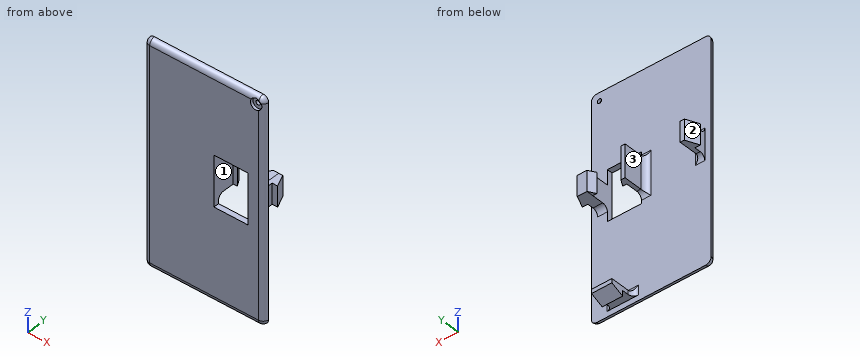
from build123d import *

# Parameters (mm, degrees)
SKETCH_1_W          = 44
SKETCH_1_H          = 81
EXTRUDE_1_DEPTH     = 2
FILLET_1_R          = 2
SKETCH_4_W          = 1.5
SKETCH_4_H          = 7.5
EXTRUDE_4_DEPTH     = 8.8
EXTRUDE_5_DEPTH     = 7.5
SKETCH_7_R          = 0.8
CUT_EXTRUDE_1_DEPTH = 8.8
SKETCH_8_R          = 2
CUT_EXTRUDE_2_DEPTH = 1
SKETCH_10_W         = 7.5
SKETCH_10_H         = 1.5
EXTRUDE_6_DEPTH     = 9
EXTRUDE_7_DEPTH     = 7.5
SKETCH_12_W         = 12.5
SKETCH_12_H         = 18.4
CUT_EXTRUDE_3_DEPTH = 7.5
SKETCH_13_W         = 2.075122626
SKETCH_13_H         = 7.498383059
EXTRUDE_8_DEPTH     = 8.8
EXTRUDE_9_DEPTH     = 7.5
SKETCH_15_W         = 1.5
SKETCH_15_H         = 12
EXTRUDE_10_DEPTH    = 8.8
EXTRUDE_11_DEPTH    = 12
FILLET_2_R          = 2


with BuildPart() as part:
    # 草图1 → 凸台-拉伸1 (new body)
    with BuildSketch(Plane(origin=(0, 0, 0), x_dir=(1, 0, 0), z_dir=(0, 1, 0))):
        with Locations((0, 2.5)):
            Rectangle(SKETCH_1_W, SKETCH_1_H)
    extrude(amount=EXTRUDE_1_DEPTH)

    # 圆角1
    fillet_1_edges = [part.edges().sort_by_distance(p)[0] for p in [
        (0, 0, -43),
        (22, 0, -2.5),
        (0, 0, 38),
        (-22, 0, -2.5),
        (-22, 1, -43),
        (22, 1, -43),
        (22, 1, 38),
        (-22, 1, 38),
    ]]
    fillet(fillet_1_edges, radius=FILLET_1_R - 0.0001)  # a hair under: the kernel refuses the full size

    # 草图4 → 凸台-拉伸4 (add)
    with BuildSketch(Plane(origin=(0, 2, 0), x_dir=(1, 0, 0), z_dir=(0, 1, 0))):
        with Locations((-18.924971335, 0)):
            Rectangle(SKETCH_4_W, SKETCH_4_H)
    extrude_4 = extrude(amount=EXTRUDE_4_DEPTH)

    # 草图6 → 凸台-拉伸5 (add)
    with BuildSketch(Plane.XY.offset(3.75)):
        Polygon((-19.674971335, 10.8), (-21.674971335, 6.2), (-19.674971335, 6.2), align=None)
    extrude_5 = extrude(amount=-EXTRUDE_5_DEPTH)

    # 镜向2: 凸台-拉伸4, 凸台-拉伸5 across plane
    add(extrude_4.mirror(Plane(origin=(0, 0, 0), x_dir=(0, 0, 1), z_dir=(1, 0, 0))))
    add(extrude_5.mirror(Plane(origin=(0, 0, 0), x_dir=(0, 0, 1), z_dir=(1, 0, 0))))

    # 草图7 → 切除-拉伸1 (cut)
    with BuildSketch(Plane.XZ):
        with Locations(Location((19, 35, 0), (0, 0, 270))):
            Circle(SKETCH_7_R)
    extrude(amount=-CUT_EXTRUDE_1_DEPTH, mode=Mode.SUBTRACT)

    # 草图8 → 切除-拉伸2 (cut)
    with BuildSketch(Plane.XZ):
        with Locations(Location((19, 35, 0), (0, 0, 270))):
            Circle(SKETCH_8_R)
    extrude(amount=-CUT_EXTRUDE_2_DEPTH, mode=Mode.SUBTRACT)

    # 草图10 → 凸台-拉伸6 (add)
    with BuildSketch(Plane(origin=(0, 2, 0), x_dir=(1, 0, 0), z_dir=(0, 1, 0))):
        with Locations((10.5, 40.25)):
            Rectangle(SKETCH_10_W, SKETCH_10_H)
    extrude(amount=EXTRUDE_6_DEPTH)

    # 草图11 → 凸台-拉伸7 (add)
    with BuildSketch(Plane(origin=(14.25, 0, 0), x_dir=(0, 0, -1), z_dir=(1, 0, 0))):
        Polygon((41, 11), (43, 6.4), (41, 6.4), align=None)
    extrude(amount=-EXTRUDE_7_DEPTH)

    # 草图12 → 切除-拉伸3 (cut)
    with BuildSketch(Plane.XZ):
        with Locations((9.849848709, 0)):
            Rectangle(SKETCH_12_W, SKETCH_12_H)
    extrude(amount=-CUT_EXTRUDE_3_DEPTH, mode=Mode.SUBTRACT)

    # 草图13 → 凸台-拉伸8 (add)
    with BuildSketch(Plane(origin=(0, 2, 0), x_dir=(1, 0, 0), z_dir=(0, 1, 0))):
        with Locations((17.137410022, 0.000808471)):
            Rectangle(SKETCH_13_W, SKETCH_13_H)
    extrude(amount=EXTRUDE_8_DEPTH)

    # 草图14 → 凸台-拉伸9 (add)
    with BuildSketch(Plane.XY.offset(3.748383059)):
        Polygon((16.099848709, 10.8), (14.599848709, 8.3), (16.099848709, 8.3), align=None)
    extrude(amount=-EXTRUDE_9_DEPTH)

    # 草图15 → 凸台-拉伸10 (add)
    with BuildSketch(Plane(origin=(0, 2, 0), x_dir=(1, 0, 0), z_dir=(0, 1, 0))):
        with Locations((2.849848709, 0)):
            Rectangle(SKETCH_15_W, SKETCH_15_H)
    extrude(amount=EXTRUDE_10_DEPTH)

    # 草图16 → 凸台-拉伸11 (add)
    with BuildSketch(Plane.XY.offset(6)):
        Polygon((3.599848709, 10.8), (5.099848709, 8.3), (3.599848709, 8.3), align=None)
    extrude(amount=-EXTRUDE_11_DEPTH)

    # 圆角2
    fillet_2_edges = [part.edges().sort_by_distance(p)[0] for p in [
        (6.75, 2, -40.25),
        (10.5, 2, -39.5),
        (14.25, 2, -40.25),
        (2.849848709, 2, -6),
        (2.099848709, 2, 0),
        (2.849848709, 2, 6),
        (-18.924971335, 2, 3.75),
        (-18.174971335, 2, 0),
        (-18.924971335, 2, -3.75),
        (17.887410022, 2, -3.75),
    ]]
    fillet(fillet_2_edges, radius=FILLET_2_R)


solid = part.part
Here's how the part is built. I have some questions about the finished solid (model axes, mm). Face numbers are marked on the shaded views. A direction names the side the tool comes from. Round coordinates to 2 decimals unless told otherwise and drop trailing zeros. Write each question's results on one line, items separated by ' | '. Start each with the question number.
(1) If I drill on probe 1 along X at (y, z) = (9.75, -2); probe 2 along Y at (x, z) = (0, 8); probe 3 along Z at (x, y) = (-19, 4.75), over which ranges is the centre line in solid material (lowest first)? Write a range as from..to.
(2) Will these pins go through, and if not, where does the flat tip stop? P1, Ø1.8, axis at x = -20, y = 6, coming from the +Z side; P2, Ø1, axis at y = 8.5, z = -7, coming from the +X side; P3, Ø2, axis at x = 2, y = 7, coming from the +Z side; P4, Ø2, axis at y = 4, z = 0.5, coming from the +X side (3 decimals).
(3) On a 3-axis mill with a long thin cutter (end or side, diameter ignored), from which of +Z, -Z, +X, -X, +Y, -Y can I reach the whole of each face in a straight line? I mean the marked faces 1, 2 and 3. Say none if no direction works.
Solved:
1) probe 1: x = -20.13..-18.17, 2.1..4.23, 15.47..20.13 | probe 2: y = 0..2 | probe 3: z = -3.75..3.75
2) P1: stops at z = 3.75 | P2: passes through | P3: stops at z = 6 | P4: stops at x = 19.675
3) face 1: -Y | face 2: +Z, -Z, -X, +Y | face 3: +Z, -Z, +Y
